Can you work these out from the model? Positions are in its coordinate system, mm. A direction names the side the tool comes from. Give positions to 0.01 mm unless a question says otherwise; leave off trailing zeros. Loops run counter-clockwise (first coordinate to the right, second up) from the corner with the lowest first, then second, coordinate; pieces in that order, holes last. Notation, with made-up numbers: (-26.75, 26) - (12.25, 26) arc R29 cw to (12.25, 62) - close; hole circle Ø6 at (57.5, -13.75). An arc over 180 degrees is marked (long way). Use a Markdown table: item, result. Add a question column.
Autodesk Inventor part; units mm, degrees
ref_plane "YZ Plane" through (0, 0, 0) normal (1, 0, 0) x (0, 1, 0)
ref_plane "XZ Plane" through (0, 0, 0) normal (0, 1, 0) x (-1, 0, 0)
ref_plane "XY Plane" through (0, 0, 0) normal (0, 0, 1) x (1, 0, 0)
sketch "스케치1" plane through (0, 0, 0) normal (0, 1, 0) x (-1, 0, 0)
  line L0 (-16, 21) -> (16, 21)
  line L1 (21, 16) -> (21, -16)
  line L2 (16, -21) -> (-16, -21)
  line L3 (-21, -16) -> (-21, 16)
  line L4 (-21, 21) -> (21, -21) construction
  line L5 (21, 21) -> (-21, -21) construction
  line L6 (16, 21) -> (21, 16)
  line L7 (21, -16) -> (16, -21)
  line L8 (-16, -21) -> (-21, -16)
  line L9 (-21, 16) -> (-16, 21)
  point P0 (0, 0)
  dimension "d0" = 42
  dimension "d1" = 42
  dimension "d2" = 5
  dimension "d3" = 5
  dimension "d4" = 5
  dimension "d5" = 5
  dimension "d6" = 5
  dimension "d7" = 5
  dimension "d8" = 5
  dimension "d9" = 5
extrude "돌출1" add sketch "스케치1" against normal blind 37
sketch "스케치2" plane through (0, 0, 0) normal (0, 1, 0) x (1, 0, 0)
  circle A0 centre (-15.5, -15.5) radius 1.5
  line L0 (0, 0) -> (-5.5004, 0) construction
  line L1 (0, 0) -> (0, 5.7427) construction
  circle A1 centre (-15.5, 15.5) radius 1.5
  circle A2 centre (15.5, -15.5) radius 1.5
  circle A3 centre (15.5, 15.5) radius 1.5
  dimension "d12" = 3
  dimension "d13" = 31
  dimension "d14" = 31
extrude "돌출2" cut sketch "스케치2" against normal blind 10
sketch "스케치3" plane through (0, 0, 0) normal (0, 1, 0) x (1, 0, 0)
  circle A0 centre (0, 0) radius 11
  dimension "d17" = 22
extrude "돌출3" add sketch "스케치3" along normal blind 2
sketch "스케치4" plane through (0, 2, 0) normal (0, 1, 0) x (1, 0, 0)
  circle A0 centre (0, 0) radius 2.5
  line L0 (-2, -3.7589) -> (-2, 6.4181)
  point P0 (-2, 1.5)
  point P1 (-2, -1.5)
  dimension "d20" = 5
  dimension "d23" = 2
extrude "돌출4" add sketch "스케치4" along normal blind 22 contours A0 L0 picked at (-0.5259, 0.206)
sketch "스케치5" plane through (0, 2, 0) normal (0, 1, 0) x (1, 0, 0)
  arc A0 (-2, -1.5) -> (-2, 1.5) centre (0, 0) ccw
  circle A1 centre (0, 0) radius 2.5
extrude "돌출5" add sketch "스케치5" along normal blind 4
equation "\"d3\" = d2"
equation "\"d4\" = d2"
equation "\"d5\" = d4"
equation "\"d6\" = d2"
equation "\"d7\" = d6"
equation "\"d8\" = d2"
equation "\"d9\" = d8"
properties part number "스텝모터 4401"
1. Will these pins go through, and if not, where does the flat tip stop? P1, Ø2.5, axis at x = 15.5, z = -16, coming from the +Y side; P2, Ø1.5, axis at y = 14.5, z = 0.5, coming from the -X side; P3, Ø2.5, axis at x = 15.5, z = -15.5, coming from the +Y side.
2. Please list where these lines run through material, in increasing order: line 1 along Z through (x, y) = (15.5, -8); line 2 along X through (y, z) = (-6, -15). Write a range as [from, to].
3. Suppose I cut it at D-D (x = -15). List the corners of the cut face in (y, z) for me, and give its area (3 significant figures).
4. If we mould it in two halves opening along Z, with no side actions, what happens to faces 3 (the face through (-16, -10, 15)), 4 (the face through (-2, 15, 0)), 5 (the face through (-19, -18, -18))? For each: released by +Z, released by -Z, zero draft, split by the parting line, or undercut.
5. Suppose I cut it at C-C (x = -3.5). List the corners of the cut face in (y, z) for me, and give its area (3 significant figures).
6. Suppose I cut it at B-B (y = -16). List the corners of the cut face in (x, z) for me.
7. On a 3-axis mill with a long thin cutter (end or side, diameter ignored), from which of +Z, -Z, +X, -X, +Y, -Y can I reach the whole of each face in a straight line? I mean faces 1 (the face through (19, -18, 18)), 2 (the face through (-9, 0, -9)). Say none if no direction works.
8. Suppose I cut it at A-A (z = 0). List the corners of the cut face in (x, y) for me.
Results below:
| question | item | result |
|---|---|---|
| 1 | P1 | y = 0 |
| 1 | P2 | x = -2 |
| 1 | P3 | y = -10 |
| 2 | line 1 | [-21, -17], [-14, 14], [17, 21] |
| 2 | line 2 | [-21, -16.91], [-14.09, 14.09], [16.91, 21] |
| 3 | outline | (-37, -21) - (0, -21) - (0, -16.91) - (-10, -16.91) - (-10, -14.09) - (0, -14.09) - (0, 14.09) - (-10, 14.09) - (-10, 16.91) - (0, 16.91) - (0, 21) - (-37, 21) - close |
| 3 | area | 1,500 mm² |
| 4 | face 3 | undercut |
| 4 | face 4 | zero draft |
| 4 | face 5 | released by -Z |
| 5 | outline | (-37, -21) - (0, -21) - (0, -10.43) - (2, -10.43) - (2, 10.43) - (0, 10.43) - (0, 21) - (-37, 21) - close |
| 5 | area | 1,600 mm² |
| 6 | outline | (-21, -16) - (-16, -21) - (16, -21) - (21, -16) - (21, 16) - (16, 21) - (-16, 21) - (-21, 16) - close |
| 7 | face 1 | +Z, +X, +Y, -Y |
| 7 | face 2 | +Y |
| 8 | outline | (-21, -37) - (21, -37) - (21, 0) - (11, 0) - (11, 2) - (2.5, 2) - (2.5, 24) - (-2, 24) - (-2, 6) - (-2.5, 6) - (-2.5, 2) - (-11, 2) - (-11, 0) - (-21, 0) - close |
